Source: CAD feature listing. Evaluate the final solid. Frame: model axes, mm. A direction names the side the tool comes from. Give positions to 0.01 mm unless a question says otherwise; leave off trailing zeros. Order: outer loops, then holes, each group sorted by start corner. A loop starts at its lowest first (then second) coordinate and runs counter-clockwise, first axis right, second up. Notation, with made-up numbers: M 60.25,2 L 75.25,2 A24 ccw 75.25,26 Z; hole C 50.5,-31.5 d4. An arc over 180 degrees is marked long. Answer as a JSON object with one key per item and string values. Group by question number.
1. Section query A-A (y = -78.5). Output: boundary loops of the cut face in (x, z).
2. Material intervals for L1, parallel to Y at x = -90.5, z = 3.5; L2, parallel to Y at x = 99, z = 1; L3, parallel to Y at x = 100, z = 4, sorted ascending. Write a range as [from, to].
3. Pull-direction query (Y, two-part tool) for faces 4 (the flat face through (-241.635, -330.744, 3.081)), 5 (the flat face through (214.25, -110, -30)), 6 (the cylindrical face through (-193.7, -95.8, 3.1)), 7 (the flat face through (179, -88.114, -30)); classes: +Y half, -Y half, draft (parallel to the pull), parting line (faces both ways), or undercut.
4. Pin query (flat end, axial travel): P1, Ø3, axis at x = 180, z = -39, coming from the -Y side; P2, Ø5, axis at y = -180, z = 2, coming from the +X side; P3, Ø1.9, axis at y = -170, z = 3.5, coming from the -X side. Return the tip coordinate at first contact, or that it passes through.
5. Section query B-B (x = -23.5). Output: boundary loops of the cut face in (y, z), plus the area to 3 significant figures.
6. Set-up query: faces 1 (the flat face through (143.75, -110, -30)), 2 (the flat face through (179, -130.614, -30)), 3 (the flat face through (77, -240.114, -30)). Return all of +Z, -Z, +X, -X, +Y, -Y with unobstructed straight access to the full face (end or side cutting, diameter ignored); none if empty.
7. Section query D-D (x = 179). Output: boundary loops of the cut face in (y, z), plus the area to 3 significant figures.
8. Section query C-C (y = -251.5). Output: boundary loops of the cut face in (x, z), plus the area to 3 significant figures.
from build123d import *

# Parameters (mm, degrees)
SKETCH1_R           = 20
SKETCH1_R_2         = 3
SKETCH1_W           = 57
SKETCH1_H           = 57
SKETCH1_W_2         = 45.5
SKETCH1_H_2         = 28.5
SKETCH1_W_3         = 29
SKETCH1_H_3         = 29
BOSS_EXTRUDE1_DEPTH = 6.25
SKETCH2_W           = 70.5
SKETCH2_H           = 42.5
SKETCH2_W_2         = 50
SKETCH2_H_2         = 33
BOSS_EXTRUDE2_DEPTH = 60


with BuildPart() as part:
    # Sketch1 → Boss-Extrude1 (new body)
    with BuildSketch(Plane.XY):
        Polygon((-340, 0), (340, 0), (340, -42), (325, -42), (325, -267), (340, -267), (340, -290), (145.985298173, -370.363520797), (-145.985298173, -370.363520797), (-340, -290), (-340, -267), (-325, -267), (-325, -42), (-340, -42), align=None)
        with Locations((-179, -109.363520797)):
            Circle(SKETCH1_R, mode=Mode.SUBTRACT)
        with Locations((179, -109.363520797)):
            Circle(SKETCH1_R, mode=Mode.SUBTRACT)
        with Locations((-99, -65)):
            Circle(SKETCH1_R_2, mode=Mode.SUBTRACT)
        with Locations((-100, -311.863520797)):
            Circle(SKETCH1_R_2, mode=Mode.SUBTRACT)
        with Locations((99, -65)):
            Circle(SKETCH1_R_2, mode=Mode.SUBTRACT)
        with Locations((100, -311.863520797)):
            Circle(SKETCH1_R_2, mode=Mode.SUBTRACT)
        with Locations((-115.5, -179.863520797)):
            Rectangle(SKETCH1_W, SKETCH1_H, mode=Mode.SUBTRACT)
        with Locations((-38.5, -179.863520797)):
            Rectangle(SKETCH1_W, SKETCH1_H, mode=Mode.SUBTRACT)
        with Locations((38.5, -179.863520797)):
            Rectangle(SKETCH1_W, SKETCH1_H, mode=Mode.SUBTRACT)
        with Locations((115.5, -179.863520797)):
            Rectangle(SKETCH1_W, SKETCH1_H, mode=Mode.SUBTRACT)
        with Locations((-77, -256.613520797)):
            Rectangle(SKETCH1_W_2, SKETCH1_H_2, mode=Mode.SUBTRACT)
        with Locations((77, -256.613520797)):
            Rectangle(SKETCH1_W_2, SKETCH1_H_2, mode=Mode.SUBTRACT)
        with Locations((0, -86.363520797)):
            Rectangle(SKETCH1_W_3, SKETCH1_H_3, mode=Mode.SUBTRACT)
    extrude(amount=BOSS_EXTRUDE1_DEPTH)

    # Sketch2 → Boss-Extrude2 (add)
    with BuildSketch(Plane.XY):
        with Locations((179, -109.363520797)):
            Rectangle(SKETCH2_W, SKETCH2_H)
        with Locations((77, -256.613520797)):
            Rectangle(SKETCH2_W_2, SKETCH2_H_2)
    extrude(amount=-BOSS_EXTRUDE2_DEPTH)


solid = part.part
Answer sheet:
{
 "1": {"outline": "M -325,0 L -14.5,0 L -14.5,6.25 L -325,6.25 Z; M 14.5,0 L 325,0 L 325,6.25 L 14.5,6.25 Z"},
 "2": {"L1": "[-370.36, -270.86], [-242.36, -208.36], [-151.36, 0]", "L2": "[-370.36, -314.69], [-309.04, -270.86], [-242.36, -208.36], [-151.36, -68], [-62, 0]", "L3": "[-370.36, -314.86], [-308.86, -208.36], [-151.36, -67.83], [-62.17, 0]"},
 "3": {"face 4": "-Y half", "face 5": "draft", "face 6": "undercut", "face 7": "+Y half"},
 "4": {"P1": "y = -130.61", "P2": "x = 325", "P3": "x = -325"},
 "5": {"outline": "M -370.36,0 L -208.36,0 L -208.36,6.25 L -370.36,6.25 Z; M -151.36,0 L 0,0 L 0,6.25 L -151.36,6.25 Z", "area": "1,960 mm^2"},
 "6": {"face 1": "-Z, -X, +Y, -Y", "face 2": "-Z, +X, -X, -Y", "face 3": "-Z, +X, -X, +Y"},
 "7": {"outline": "M -356.69,0 L -130.61,0 L -130.61,-60 L -88.11,-60 L -88.11,0 L 0,0 L 0,6.25 L -89.36,6.25 L -89.36,0 L -129.36,0 L -129.36,6.25 L -356.69,6.25 Z", "area": "4,530 mm^2"},
 "8": {"outline": "M -325,0 L -99.75,0 L -99.75,6.25 L -325,6.25 Z; M -54.25,0 L 52,0 L 52,-60 L 102,-60 L 102,0 L 325,0 L 325,6.25 L 99.75,6.25 L 99.75,0 L 54.25,0 L 54.25,6.25 L -54.25,6.25 Z", "area": "6,490 mm^2"}
}
